Read the model definition and answer for the solid it produces. Units are mm, in the model's axes. Coordinates: 2 decimals unless noted, no trailing zeros. Write each loop counter-clockwise with the first axis right and the second up, starting at its lowest first coordinate (ties: lowest second). Pieces come first, ordered by that corner, then holes. Notation, with made-up numbers: (72, -2.75) -> (117, -2.75) arc R32 ccw to (117, 31.25) -> close; hole circle Ø11 at (-0.75, 29.25). An arc over 180 degrees is marked (long way). Return JSON: item names as keys, results as strings.
from build123d import *

# Parameters (mm, degrees)
SKETCH1_W            = 189.35
SKETCH1_H            = 1094.236516537
BOSS_EXTRUDE1_DEPTH  = 18
CAVITY1_START        = -84.195551816
CAVITY1_OUTLINE_W    = 18
CAVITY1_OUTLINE_H    = 18
CAVITY1_DEPTH        = 30
CAVITY1_START_2      = 117.922706453
CAVITY1_2_OUTLINE_W  = 18
CAVITY1_2_OUTLINE_H  = 18
CAVITY1_2_DEPTH      = 30
CAVITY1_START_3      = 347.922706453
CAVITY1_3_OUTLINE_W  = 18
CAVITY1_3_OUTLINE_H  = 18
CAVITY1_3_DEPTH      = 30
CAVITY1_START_4      = 577.922706453
CAVITY1_4_OUTLINE_W  = 18
CAVITY1_4_OUTLINE_H  = 18
CAVITY1_4_DEPTH      = 30
CAVITY1_START_5      = 780.040964722
CAVITY1_5_OUTLINE_W  = 18
CAVITY1_5_OUTLINE_H  = 18
CAVITY1_5_DEPTH      = 30
SKETCH2_W            = 79.675
SKETCH2_H            = 18
CUT_EXTRUDE1_DEPTH   = 18
SKETCH3_R            = 39.700513166
CUT_EXTRUDE2_DEPTH   = 18
M3_CLEARANCE_HOLE1_D = 3.4
SKETCH7_R            = 3
CUT_EXTRUDE3_DEPTH   = 20


# Read off the part's stored shape, not the designer's step: Cavity1
with BuildPart() as part:
    # Sketch1 → Boss-Extrude1 (new body)
    with BuildSketch(Plane.XY):
        with Locations((76.675, 362.922706452)):
            Rectangle(SKETCH1_W, SKETCH1_H)
    extrude(amount=BOSS_EXTRUDE1_DEPTH)

    # Cavity1 outline → Cavity1 (cut)
    with BuildSketch(Plane(origin=(0, 0, 0), x_dir=(1, 0, 0), z_dir=(0, 1, 0)).offset(CAVITY1_START)):
        with Locations((-9, -9)):
            Rectangle(CAVITY1_OUTLINE_W, CAVITY1_OUTLINE_H)
    extrude(amount=CAVITY1_DEPTH, mode=Mode.SUBTRACT)

    # Cavity1 2 outline → Cavity1 2 (cut)
    with BuildSketch(Plane(origin=(0, 0, 0), x_dir=(1, 0, 0), z_dir=(0, 1, 0)).offset(CAVITY1_START_2)):
        with Locations((-9, -9)):
            Rectangle(CAVITY1_2_OUTLINE_W, CAVITY1_2_OUTLINE_H)
    extrude(amount=CAVITY1_2_DEPTH, mode=Mode.SUBTRACT)

    # Cavity1 3 outline → Cavity1 3 (cut)
    with BuildSketch(Plane(origin=(0, 0, 0), x_dir=(1, 0, 0), z_dir=(0, 1, 0)).offset(CAVITY1_START_3)):
        with Locations((-9, -9)):
            Rectangle(CAVITY1_3_OUTLINE_W, CAVITY1_3_OUTLINE_H)
    extrude(amount=CAVITY1_3_DEPTH, mode=Mode.SUBTRACT)

    # Cavity1 4 outline → Cavity1 4 (cut)
    with BuildSketch(Plane(origin=(0, 0, 0), x_dir=(1, 0, 0), z_dir=(0, 1, 0)).offset(CAVITY1_START_4)):
        with Locations((-9, -9)):
            Rectangle(CAVITY1_4_OUTLINE_W, CAVITY1_4_OUTLINE_H)
    extrude(amount=CAVITY1_4_DEPTH, mode=Mode.SUBTRACT)

    # Cavity1 5 outline → Cavity1 5 (cut)
    with BuildSketch(Plane(origin=(0, 0, 0), x_dir=(1, 0, 0), z_dir=(0, 1, 0)).offset(CAVITY1_START_5)):
        with Locations((-9, -9)):
            Rectangle(CAVITY1_5_OUTLINE_W, CAVITY1_5_OUTLINE_H)
    extrude(amount=CAVITY1_5_DEPTH, mode=Mode.SUBTRACT)

    # Sketch2 → Cut-Extrude1 (cut)
    with BuildSketch(Plane.XY.offset(18)):
        with Locations((21.8375, -175.195551816)):
            Rectangle(SKETCH2_W, SKETCH2_H)
        with Locations((131.5125, -175.195551816)):
            Rectangle(SKETCH2_W, SKETCH2_H)
        with Locations((21.8375, 901.040964721)):
            Rectangle(SKETCH2_W, SKETCH2_H)
        with Locations((131.5125, 901.040964721)):
            Rectangle(SKETCH2_W, SKETCH2_H)
    extrude(amount=-CUT_EXTRUDE1_DEPTH, mode=Mode.SUBTRACT)

    # Sketch3 → Cut-Extrude2 (cut)
    with BuildSketch(Plane.XY.offset(18)):
        with Locations((77.75, 773.505430817)):
            Circle(SKETCH3_R)
    extrude(amount=-CUT_EXTRUDE2_DEPTH, mode=Mode.SUBTRACT)

    # M3 Clearance Hole1 (through all)
    with Locations(Plane.XY.offset(18)):
        with Locations((-9, 851.040964721), (-9, -125.195551816), (-9, 477.922706453), (-9, 247.922706453), (76.675, 901.040964721), (76.675, -175.195551816)):
            Hole(M3_CLEARANCE_HOLE1_D / 2)

    # Sketch7 → Cut-Extrude3 (cut)
    with BuildSketch(Plane(origin=(0, 0, 0), x_dir=(-1, 0, 0), z_dir=(0, 0, -1))):
        with Locations((2.121320344, -56.31687216)):
            Circle(SKETCH7_R)
        with Locations((2.121320344, -82.074231473)):
            Circle(SKETCH7_R)
        with Locations((2.121320344, 145.80312784)):
            Circle(SKETCH7_R)
        with Locations((2.121320344, 120.045768527)):
            Circle(SKETCH7_R)
        with Locations((2.121320344, 605.799644378)):
            Circle(SKETCH7_R)
        with Locations((2.121320344, 580.042285065)):
            Circle(SKETCH7_R)
        with Locations((2.121320344, 807.919644378)):
            Circle(SKETCH7_R)
        with Locations((2.121320344, 782.162285065)):
            Circle(SKETCH7_R)
        with Locations((2.121320344, 375.801386109)):
            Circle(SKETCH7_R)
        with Locations((2.121320344, 350.044026796)):
            Circle(SKETCH7_R)
        with Locations((-59.553679656, -168.31687216)):
            Circle(SKETCH7_R)
        with Locations((-93.796320344, -168.31687216)):
            Circle(SKETCH7_R)
        with Locations((-93.796320344, 894.162285065)):
            Circle(SKETCH7_R)
        with Locations((-59.553679656, 894.162285065)):
            Circle(SKETCH7_R)
    extrude(amount=-CUT_EXTRUDE3_DEPTH, mode=Mode.SUBTRACT)


solid = part.part
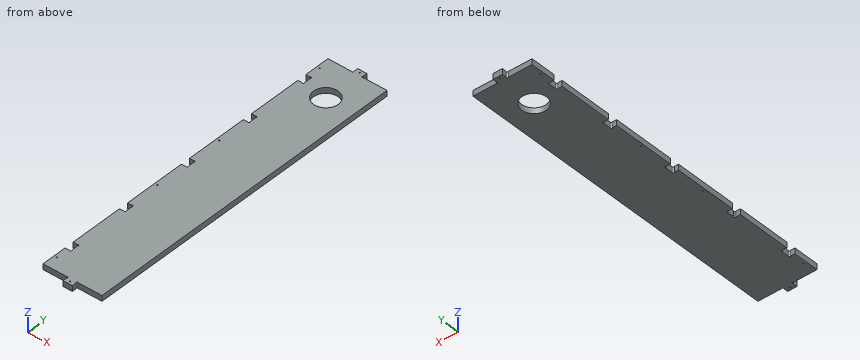
1. The part is cut by section B-B (z = 3.25). Count the separate pieces of the cut face and the enclosed holes in it, then the cut area to 3 significant figures.
Taken from the geometry:
{"separate pieces": "1", "enclosed holes": "7", "area": "194,000 mm2"}
2. Flat-ended cylindrical pins translate along their axes: pin 1 Ø4 at (x, z) = (-11.5, 13) entering from -Y; pin 2 Ø8 at (x, y) = (66, 466) entering from -Z; pin 3 Ø4 at (y, z) = (902, 10) entering from -X (3 decimals); pin 4 Ø2.5 at (x, y) = (76.68, -175.2) entering from +Z. Find the tip coordinate at first contact, or state that the pin passes through.
Taken from the geometry:
{"pin 1": "stops at y = -166.2", "pin 2": "stops at z = 0", "pin 3": "stops at x = 61.675", "pin 4": "passes through"}
3. The part is cut by section A-A (x = 12). Determine the outline of the cut face in (y, z).
Taken from the geometry:
{"outline": "(-166.2, 0) -> (892.04, 0) -> (892.04, 18) -> (-166.2, 18) -> close"}
4. Consider L1, parallel to Y at x = 79.5, z = 11.5; L2, parallel to X at y = 771, z = 13; L3, parallel to Y at x = 35, z = 9.25. Determine where each line is inside the solid, lowest interval first.
Taken from the geometry:
{"L1": "y = -184.2 to 733.84, 813.17 to 910.04", "L2": "x = -18 to 38.13, 117.37 to 171.35", "L3": "y = -166.2 to 892.04"}
